Could you check a few things on this model? Use its own coordinates, in mm. A direction names the side the tool comes from. Round coordinates to 2 decimals unless told otherwise and drop trailing zeros. Order: outer loops, then holes, each group sorted by start corner. A loop starts at its lowest first (then second) coordinate and runs counter-clockwise, first axis right, second up. Notation, with made-up numbers: M 27.5,24 L 74.5,24 A15 ccw 74.5,29 Z; hole C -31,-30 d9. An arc over 180 degrees is marked long. Write each question's results on one line, items separated by ' | '. Start each with the question number.
1. I'm going to push flat-ended pins straight in: pin 1 (1 mm diameter, centred on x = -49.5, z = -8, fed in from -Y); pin 2 (1 mm diameter, centred on x = 23.5, y = -0.5, fed in from +Z); pin 3 (2 mm diameter, centred on x = 42, y = -3, fed in from -Z). Where does each tip first touch, or does it pass through?
2. Please list where these lines run through material, in increasing order: L1, parallel to X at y = -0.75, z = 3; L2, parallel to X at y = -2.85, z = 44.5; L3, parallel to Y at x = 9, z = 21.
3. Suppose I cut it at A-A on z = 17. Write out the boundary of the cut face in (x, y) (3 decimals).
4. For faces 4 (the flat face through (-22, -3.81, 13)), 5 (the cylindrical face through (43.226, -2.325, 11.872)), 6 (the flat face through (-81.956, -2, 17)), which set-ups out of +Z, -Z, +X, -X, +Y, -Y let a thin tool reach every point of the face, with its end or its side?
5. Suppose I cut it at B-B on z = 30.5. Write out the boundary of the cut face in (x, y), and give its area (3 significant figures).
6. We'd pull the mould along Z, two halves only. Please class faces 1 (the cylindrical face through (-22.384, -0.738, 47.761)), 2 (the flat face through (-22, 0, 13)), 3 (the flat face through (-80.524, -2, 17)): released by +Z, released by -Z, zero draft, split by the parting line, or undercut.
7. Suppose I cut it at D-D on z = -3. Write out the boundary of the cut face in (x, y) (3 decimals), and give its area (3 significant figures).
8. Suppose I cut it at C-C on x = -14.5. Write out the boundary of the cut face in (y, z), and give its area (3 significant figures).
from build123d import *

# Parameters (mm, degrees)
F0_W          = 123.7234
F0_H          = 72.7202
F1_DEPTH      = 3.81
F2_R          = 2.159
F2_R_2        = 1.397
F3_DEPTH      = 72.7202
F4_R          = 1.397
F5_DEPTH      = 20.066
F6_R          = 1.397
F7_DEPTH      = 20.066
F8_W          = 1.4323815703
F8_H          = 3.1365510076
F9_DEPTH      = 25.4
F10_T1_DEPTH  = 135.9876048969
F10_T3_DEPTH  = 84.9844048969
F10_T8_DEPTH  = 84.9844048969
F10_S10_R     = 2.159
F10_T11_DEPTH = 44
F10_T15_DEPTH = 84.9844048969
F10_S17_R     = 2.159
F10_T18_DEPTH = 44
F10_T22_DEPTH = 84.9844048969
F10_S24_R     = 2.159
F10_T25_DEPTH = 44
F10_T30_DEPTH = 84.9844048969
F10_S31_R     = 2.159
F10_T32_DEPTH = 44
F10_T37_DEPTH = 84.9844048969
F10_S38_R     = 2.159
F10_T39_DEPTH = 44


# Not quite as in the source:
# - a fillet or chamfer that OpenCascade refuses, or shapes differently, is made with other operations: its cross-section is extruded or revolved along the edge and cut away or added


with BuildPart() as f1:
    # F0 (on Front) → F1 (new body)
    with BuildSketch(Plane.XZ):
        with Locations((-21.517843008, 12.1004326615)):
            Rectangle(F0_W, F0_H)
    extrude(amount=F1_DEPTH)

    # F2 (on face) → F3 (join)
    with BuildSketch(Plane(origin=(0, 0, -24.2596673385), x_dir=(1, 0, 0), z_dir=(0, 0, -1))):
        with Locations((41.893256992, 1.905)):
            Circle(F2_R)
        with Locations((41.893256992, 1.905)):
            Circle(F2_R_2, mode=Mode.SUBTRACT)
    extrude(amount=-F3_DEPTH)

    # F4 (on face) → F5 (cut)
    with BuildSketch(Plane(origin=(0, 0, -24.2596673385), x_dir=(1, 0, 0), z_dir=(0, 0, -1))):
        with BuildLine():
            ThreePointArc((40.343856992, 0.4014573036), (44.052256992, 1.905), (40.343856992, 3.4085426964))
            Line((40.343856992, 3.4085426964), (40.343856992, 0.4014573036))
        make_face()
        with Locations((41.893256992, 1.905)):
            Circle(F4_R, mode=Mode.SUBTRACT)
    extrude(amount=-F5_DEPTH, mode=Mode.SUBTRACT)

    # F6 (on face) → F7 (cut)
    with BuildSketch(Plane.XY.offset(48.4605326615)):
        with BuildLine():
            ThreePointArc((40.343856992, -3.4085426964), (44.052256992, -1.905), (40.343856992, -0.4014573036))
            Line((40.343856992, -0.4014573036), (40.343856992, -3.4085426964))
        make_face()
        with Locations((41.893256992, -1.905)):
            Circle(F6_R, mode=Mode.SUBTRACT)
    extrude(amount=-F7_DEPTH, mode=Mode.SUBTRACT)

    # F8 (on face) → F9 (cut)
    with BuildSketch(Plane(origin=(0, 0, 0), x_dir=(-1, 0, 0), z_dir=(0, 1, 0))):
        with Locations((81.2400989234, 17.0341590419)):
            Rectangle(F8_W, F8_H)
    extrude(amount=-F9_DEPTH, mode=Mode.SUBTRACT)

    # F10: fillet of radius 2.4528409794 on 4 edges, made by hand

    # F10_s2 → F10_t1 (cut)
    with BuildSketch(Plane.YZ.offset(-89.5116454565)):
        with BuildLine():
            ThreePointArc((-2.4528409794, 48.4605326615), (-0.7184204897, 47.7421121718), (0, 46.0076916821))
            Line((0, 46.0076916821), (0, 48.4605326615))
            Line((0, 48.4605326615), (-2.4528409794, 48.4605326615))
        make_face()
        with BuildLine():
            ThreePointArc((-2.4528409794, -24.2596673385), (-0.7184204897, -23.5412468488), (0, -21.8068263591))
            Line((0, -21.8068263591), (0, -24.2596673385))
            Line((0, -24.2596673385), (-2.4528409794, -24.2596673385))
        make_face()
    extrude(amount=F10_T1_DEPTH, mode=Mode.SUBTRACT)

    # F10_s4 → F10_t3 (cut)
    with BuildSketch(Plane.XY.offset(-30.3917697869)):
        with BuildLine():
            ThreePointArc((-83.379543008, -2.4528409794), (-82.6611225184, -0.7184204897), (-80.9267020287, 0))
            Line((-80.9267020287, 0), (-83.379543008, 0))
            Line((-83.379543008, 0), (-83.379543008, -2.4528409794))
        make_face()
    extrude(amount=F10_T3_DEPTH, mode=Mode.SUBTRACT)


with BuildPart() as f10_tool6:
    # F10_s7 → F10_t8 (new body)
    with BuildSketch(Plane.XY.offset(-30.3917697869)):
        with BuildLine():
            ThreePointArc((37.8910160126, 0), (39.6254365023, -0.7184204897), (40.343856992, -2.4528409794))
            Line((40.343856992, -2.4528409794), (40.343856992, 0))
            Line((40.343856992, 0), (37.8910160126, 0))
        make_face()
    extrude(amount=F10_T8_DEPTH)

    split(bisect_by=Plane.XY.offset(-4.1936673385), keep=Keep.BOTTOM)

    # F10_s10 → F10_t11 (cut, symmetric)
    with BuildSketch(Plane.XY.offset(12.1)):
        with Locations((41.893256992, -1.905)):
            Circle(F10_S10_R)
    extrude(amount=F10_T11_DEPTH, both=True, mode=Mode.SUBTRACT)


with BuildPart() as f1_1:
    add(f1.part)

    # F10_t5: cut F10_tool6
    add(f10_tool6.part, mode=Mode.SUBTRACT)


with BuildPart() as f10_tool13:
    # F10_s14 → F10_t15 (new body)
    with BuildSketch(Plane.XY.offset(-30.3917697869)):
        with BuildLine():
            ThreePointArc((37.8910160126, 0), (39.6254365023, -0.7184204897), (40.343856992, -2.4528409794))
            Line((40.343856992, -2.4528409794), (40.343856992, 0))
            Line((40.343856992, 0), (37.8910160126, 0))
        make_face()
    extrude(amount=F10_T15_DEPTH)

    split(bisect_by=Plane.XY.offset(-4.1936673385), keep=Keep.BOTTOM)

    # F10_s17 → F10_t18 (intersect, symmetric)
    with BuildSketch(Plane.XY.offset(12.1)):
        with Locations((41.893256992, -1.905)):
            Circle(F10_S17_R)
    extrude(amount=F10_T18_DEPTH, both=True, mode=Mode.INTERSECT)


with BuildPart() as f1_2:
    add(f1_1.part)

    # F10_t12: cut F10_tool13
    add(f10_tool13.part, mode=Mode.SUBTRACT)


with BuildPart() as f10_tool20:
    # F10_s21 → F10_t22 (new body)
    with BuildSketch(Plane.XY.offset(-30.3917697869)):
        with BuildLine():
            ThreePointArc((37.8910160126, 0), (39.6254365023, -0.7184204897), (40.343856992, -2.4528409794))
            Line((40.343856992, -2.4528409794), (40.343856992, 0))
            Line((40.343856992, 0), (37.8910160126, 0))
        make_face()
    extrude(amount=F10_T22_DEPTH)

    split(bisect_by=Plane.XY.offset(-4.1936673385), keep=Keep.TOP)

    # F10_s24 → F10_t25 (cut, symmetric)
    with BuildSketch(Plane.XY.offset(12.1)):
        with Locations((41.893256992, -1.905)):
            Circle(F10_S24_R)
    extrude(amount=F10_T25_DEPTH, both=True, mode=Mode.SUBTRACT)

    split(bisect_by=Plane.XY.offset(28.3945326615), keep=Keep.BOTTOM)


with BuildPart() as f1_3:
    add(f1_2.part)

    # F10_t19: cut F10_tool20
    add(f10_tool20.part, mode=Mode.SUBTRACT)


with BuildPart() as f10_tool28:
    # F10_s29 → F10_t30 (new body)
    with BuildSketch(Plane.XY.offset(-30.3917697869)):
        with BuildLine():
            ThreePointArc((37.8910160126, 0), (39.6254365023, -0.7184204897), (40.343856992, -2.4528409794))
            Line((40.343856992, -2.4528409794), (40.343856992, 0))
            Line((40.343856992, 0), (37.8910160126, 0))
        make_face()
    extrude(amount=F10_T30_DEPTH)

    # F10_s31 → F10_t32 (cut, symmetric)
    with BuildSketch(Plane.XY.offset(12.1)):
        with Locations((41.893256992, -1.905)):
            Circle(F10_S31_R)
    extrude(amount=F10_T32_DEPTH, both=True, mode=Mode.SUBTRACT)

    split(bisect_by=Plane.XY.offset(28.3945326615), keep=Keep.TOP)


with BuildPart() as f1_4:
    add(f1_3.part)

    # F10_t27: cut F10_tool28
    add(f10_tool28.part, mode=Mode.SUBTRACT)


with BuildPart() as f10_tool35:
    # F10_s36 → F10_t37 (new body)
    with BuildSketch(Plane.XY.offset(-30.3917697869)):
        with BuildLine():
            ThreePointArc((37.8910160126, 0), (39.6254365023, -0.7184204897), (40.343856992, -2.4528409794))
            Line((40.343856992, -2.4528409794), (40.343856992, 0))
            Line((40.343856992, 0), (37.8910160126, 0))
        make_face()
    extrude(amount=F10_T37_DEPTH)

    # F10_s38 → F10_t39 (intersect, symmetric)
    with BuildSketch(Plane.XY.offset(12.1)):
        with Locations((41.893256992, -1.905)):
            Circle(F10_S38_R)
    extrude(amount=F10_T39_DEPTH, both=True, mode=Mode.INTERSECT)

    split(bisect_by=Plane.XY.offset(28.3945326615), keep=Keep.TOP)


with BuildPart() as f1_5:
    add(f1_4.part)

    # F10_t34: cut F10_tool35
    add(f10_tool35.part, mode=Mode.SUBTRACT)


solid = f1_5.part
Filled sheet:
1) pin 1: stops at y = -3.81 | pin 2: stops at z = 47.98 | pin 3: stops at z = -4.19
2) L1: x = -82.69 to 39.66, 40.07 to 41.11, 42.68 to 43.72 | L2: x = -83.38 to 40.34 | L3: y = -3.81 to 0
3) outline: M -83.38,-3.81 L -81.956,-3.81 L -81.956,-0.227 A2.453 ccw -83.38,-2.453 Z; M -80.524,-3.81 L 40.344,-3.81 L 40.344,-3.409 A2.159 ccw long 39.908,-1.057 A2.453 ccw 37.891,0 L -80.524,0 Z; hole C 41.893,-1.905 d2.794
4) face 4: +Z, -Z, -X, -Y | face 5: +Z, -Z | face 6: +Y, -Y
5) outline: M -83.38,-3.81 L 40.34,-3.81 L 40.34,-2.45 A2.45 ccw 37.89,0 L -80.93,0 A2.45 ccw -83.38,-2.45 Z | area: 469 mm^2
6) face 1: released by +Z | face 2: zero draft | face 3: undercut
7) outline: M -83.38,-3.81 L 40.344,-3.81 L 40.344,-3.409 A2.159 ccw long 39.908,-1.057 A2.453 ccw 37.891,0 L -80.927,0 A2.453 ccw -83.38,-2.453 Z; hole C 41.893,-1.905 d2.794 | area: 476 mm^2
8) outline: M -3.81,-24.26 L -2.45,-24.26 A2.45 ccw 0,-21.81 L 0,46.01 A2.45 ccw -2.45,48.46 L -3.81,48.46 Z | area: 274 mm^2
